The model under review builds one solid part; all positions refer to its coordinate system, in mm. A direction names the side the tool comes from. Give positions to 0.01 mm unless a question says otherwise; leave off trailing zeros. Order: outer loops, then holes, each group sorted by start corner. A loop starts at its lowest first (then second) coordinate and runs counter-clockwise, first axis right, second up. Notation, with made-up numbers: M 32,85 L 68,85 A11 ccw 68,102 Z; hole C 49.25,19.25 d10. An arc over 180 degrees is marked long. One line per question, with ' | ' between items. Start each with the question number.
1. Insertion check: P1, Ø1.5, axis at x = -1, y = 43.5, coming from the -Z side; P2, Ø1, axis at y = 33, z = -2.5, coming from the +X side; P3, Ø2, axis at y = 8.5, z = -1, coming from the -X side (3 decimals). Each pin has a flat end and moves straight along its axis. Give the tip position at first contact, or say it passes through.
2. We need section A-A on y = 56. Write out the cut boundary in (x, z) (3 decimals), then the cut area to 3 significant figures.
3. For faces 1 (the face through (-3.2, 0, -1.1)), 2 (the face through (4.762, -2, 0)), list the 3-axis set-ups (+Z, -Z, +X, -X, +Y, -Y) from which the entire face can be reached by the end or side of a thin tool; tool diameter is ignored.
4. Wall thickness on L1, parallel to Y at x = 0.75, z = -4; L2, parallel to Z at x = 0, y = 32.5 (3 decimals); L3, parallel to X at y = 79, z = 0.25: over which ranges is each line inside the solid? List them lowest first.
```python
from build123d import *

# Parameters (mm, degrees)
F2_R     = 3.175
F3_DEPTH = 88.9
F5_DEPTH = 4.7625
F6_SIZE  = 0.635


# Not quite as in the source:
# - a length typed as a fraction of an inch, garbled in the dataset ("3 / 203.2 mm" for 3/8 in), is restored


with BuildPart() as f3:
    # F2 (on Front) → F3 (new body)
    with BuildSketch(Plane.XZ):
        Circle(F2_R)
    extrude(amount=-F3_DEPTH)

    # F4 (on Front) → F5 (join)
    with BuildSketch(Plane.XZ):
        Polygon((0, -5.499261314), (4.7625, -2.749630657), (4.7625, 2.749630657), (0, 5.499261314), (-4.7625, 2.749630657), (-4.7625, -2.749630657), align=None)
    extrude(amount=F5_DEPTH)

    # F6
    f6_edges = [f3.edges().sort_by_distance(p)[0] for p in [
        (-3.175, 88.9, 0),
    ]]
    chamfer(f6_edges, length=F6_SIZE)

    # F7 (on Top) → F8 (revolve, cut)
    with BuildSketch(Plane.XY):
        Polygon((11.8464599431, -4.7625), (11.8464599431, -0.6725738199), (4.7625, -4.7625), align=None)
    revolve(axis=Axis((0, -2.38125, 0), (0, -1, 0)), mode=Mode.SUBTRACT)


solid = f3.part
```
Entries:
1) P1: stops at z = -3.17 | P2: stops at x = 2.47 | P3: stops at x = -3.175
2) outline: C 0,0 d6.35 | area: 31.7 mm^2
3) face 1: +Y | face 2: +Z, -Z, +X, +Y, -Y
4) L1: y = -4.76 to 0 | L2: z = -3.175 to 3.175 | L3: x = -3.17 to 3.17
